```python
from build123d import *

# Parameters (mm, degrees)
BOSS_EXTRUDE2_DEPTH = 15
SKETCH5_R           = 1.5
CUT_EXTRUDE3_DEPTH  = 8
BOSS_EXTRUDE4_DEPTH = 5.5
CUT_EXTRUDE4_DEPTH  = 10
CUT_EXTRUDE5_DEPTH  = 7
SKETCH5_4_R         = 1.5
CUT_EXTRUDE6_DEPTH  = 10
SKETCH10_W          = 5.6
SKETCH10_H          = 2.4
SKETCH10_W_2        = 5.5
CUT_EXTRUDE7_DEPTH  = 24
SKETCH10_3_W        = 5.6
SKETCH10_3_H        = 2.4
SKETCH10_3_W_2      = 5.5
BOSS_EXTRUDE5_DEPTH = 4.2


with BuildPart() as part:
    # Sketch3 → Boss-Extrude2 (new body)
    with BuildSketch(Plane.XY):
        Polygon((380.706426849, -77.512840587), (380.706426849, -131.012840587), (354.706426849, -131.012840587), (337.706426849, -77.512840587), align=None)
    extrude(amount=BOSS_EXTRUDE2_DEPTH)

    # Sketch5 → Cut-Extrude3 (cut)
    with BuildSketch(Plane(origin=(0, -77.512840587, 0), x_dir=(1, 0, 0), z_dir=(0, 1, 0))):
        with Locations(Location((344.406426849, -7.5, 0), (0, 0, 270))):
            Circle(SKETCH5_R)
        with Locations(Location((359.406426849, -7.5, 0), (0, 0, 270))):
            Circle(SKETCH5_R)
        with Locations(Location((374.406426849, -7.5, 0), (0, 0, 270))):
            Circle(SKETCH5_R)
    extrude(amount=-CUT_EXTRUDE3_DEPTH, mode=Mode.SUBTRACT)

    # Sketch7 → Boss-Extrude4 (add)
    with BuildSketch(Plane(origin=(0, 0, 0), x_dir=(-1, 0, 0), z_dir=(0, 0, -1))):
        Polygon((-380.706426849, -77.512840587), (-337.706426849, -77.512840587), (-354.706426849, -131.012840587), (-380.706426849, -131.012840587), align=None)
    extrude(amount=BOSS_EXTRUDE4_DEPTH)

    # Sketch8 → Cut-Extrude4 (cut)
    with BuildSketch(Plane(origin=(380.706426849, 0, 0), x_dir=(0, 0, -1), z_dir=(1, 0, 0))):
        with BuildLine():
            ThreePointArc((-3.25, -98.312840587), (-3.689339828, -97.252180415), (-4.75, -96.812840587))
            Line((-4.75, -96.812840587), (-4.75, -99.812840587))
            ThreePointArc((-4.75, -99.812840587), (-3.689339828, -99.373500759), (-3.25, -98.312840587))
        make_face()
        with BuildLine():
            Line((-4.75, -99.812840587), (-4.75, -96.812840587))
            ThreePointArc((-4.75, -96.812840587), (-6.25, -98.312840587), (-4.75, -99.812840587))
        make_face()
        with BuildLine():
            ThreePointArc((-3.25, -122.312840587), (-3.689339828, -121.252180415), (-4.75, -120.812840587))
            Line((-4.75, -120.812840587), (-4.75, -123.812840587))
            ThreePointArc((-4.75, -123.812840587), (-3.689339828, -123.373500759), (-3.25, -122.312840587))
        make_face()
        with BuildLine():
            Line((-4.75, -123.812840587), (-4.75, -120.812840587))
            ThreePointArc((-4.75, -120.812840587), (-6.25, -122.312840587), (-4.75, -123.812840587))
        make_face()
    extrude(amount=-CUT_EXTRUDE4_DEPTH, mode=Mode.SUBTRACT)

    # Sketch9 → Cut-Extrude5 (cut)
    with BuildSketch(Plane(origin=(0, -131.012840587, 0), x_dir=(-1, 0, 0), z_dir=(0, -1, 0))):
        with BuildLine():
            ThreePointArc((-375.206426849, -4.75), (-373.706426849, -6.25), (-372.206426849, -4.75))
            Line((-372.206426849, -4.75), (-375.206426849, -4.75))
        make_face()
        with BuildLine():
            Line((-375.206426849, -4.75), (-372.206426849, -4.75))
            ThreePointArc((-372.206426849, -4.75), (-373.706426849, -3.25), (-375.206426849, -4.75))
        make_face()
        with BuildLine():
            ThreePointArc((-363.206426849, -4.75), (-361.706426849, -6.25), (-360.206426849, -4.75))
            Line((-360.206426849, -4.75), (-363.206426849, -4.75))
        make_face()
        with BuildLine():
            Line((-363.206426849, -4.75), (-360.206426849, -4.75))
            ThreePointArc((-360.206426849, -4.75), (-361.706426849, -3.25), (-363.206426849, -4.75))
        make_face()
    extrude(amount=-CUT_EXTRUDE5_DEPTH, mode=Mode.SUBTRACT)

    # Sketch5_4 → Cut-Extrude6 (cut)
    with BuildSketch(Plane(origin=(0, -77.512840587, 0), x_dir=(1, 0, 0), z_dir=(0, 1, 0))):
        with Locations(Location((359.406426849, -7.5, 0), (0, 0, 270))):
            Circle(SKETCH5_4_R)
        with Locations(Location((374.406426849, -7.5, 0), (0, 0, 270))):
            Circle(SKETCH5_4_R)
    extrude(amount=-CUT_EXTRUDE6_DEPTH, mode=Mode.SUBTRACT)

    # Sketch10 → Cut-Extrude7 (cut)
    with BuildSketch(Plane.XY.offset(15)):
        with Locations((359.312441298, -85.248108343)):
            Rectangle(SKETCH10_W, SKETCH10_H)
        with Locations((374.333669077, -85.248108343)):
            Rectangle(SKETCH10_W_2, SKETCH10_H)
    extrude(amount=-CUT_EXTRUDE7_DEPTH, mode=Mode.SUBTRACT)

    # Sketch10_3 → Boss-Extrude5 (add)
    with BuildSketch(Plane.XY.offset(15)):
        with Locations((359.312441298, -85.248108343)):
            Rectangle(SKETCH10_3_W, SKETCH10_3_H)
        with Locations((374.333669077, -85.248108343)):
            Rectangle(SKETCH10_3_W_2, SKETCH10_3_H)
    extrude(amount=-BOSS_EXTRUDE5_DEPTH)


solid = part.part
```
Geometry: final body of the model. Coordinates: model frame, mm. A direction names the side the tool comes from. Give positions to 0.01 mm unless a question says otherwise; leave off trailing zeros. Order: outer loops, then holes, each group sorted by start corner. A loop starts at its lowest first (then second) coordinate and runs counter-clockwise, first axis right, second up. Notation, with made-up numbers: M 35.5,40.25 L 46.5,40.25 A18 cw 46.5,49.25 Z; hole C 72.25,16.25 d9. An arc over 180 degrees is marked long. Answer as CSV lines item,"result". Start each with the question number.
1) Line query: line 1 (Y direction, x = 359, z = 10.5); line 2 (X direction, y = -126.25, z = 4.75); line 3 (X direction, y = -83, z = 7.5). Output: solid intervals per line, ascending. Write a range as from..to.
2) First-contact query: P1, Ø0.9, axis at x = 374, z = 5, coming from the -Y side. Flat tip, straight axial feed; report the tip coordinate or a pass-through.
3) Cut plane B-B (x = 376.5). Output: boundary loops of the cut face in (y, z).
4) Set-up query: faces 4 (the flat face through (344, -85.513, 7)), 5 (the cylindrical face through (375.205, -127.562, 4.684)), 6 (the flat face through (362.112, -85, 3)), 7 (the flat face through (370.706, -122, 5)). Return all of +Z, -Z, +X, -X, +Y, -Y with unobstructed straight access to the full face (end or side cutting, diameter ignored); none if empty.
5) Mould query, pull axis X, two halves, no side actions, for faces 1 (the flat face through (368, -131.013, 5)), 2 (the flat face through (370.706, -98, 5)), 3 (the cylindrical face through (372.942, -80.735, 7.175)). Classes: +X half, -X half, draft (parallel to the pull), parting line (faces both ways), or undercut.
6) Cut plane A-A (z = 0.5). Output: boundary loops of the cut face in (x, y), then the cut area to 3 significant figures.
7) Cut plane C-C (y = -81.5). Output: boundary loops of the cut face in (x, z), then the cut area to 3 significant figures.
Findings below:
1,line 1,"y = -131.01..-86.45, -84.05..-77.51"
1,line 2,"x = 353.19..360.21, 363.21..372.21, 375.21..380.71"
1,line 3,"x = 339.45..342.91, 345.91..357.91, 360.91..372.91, 375.91..380.71"
2,P1,"stops at y = -124.01"
3,outline,"M -131.01,-5.5 L -86.45,-5.5 L -86.45,10.8 L -84.05,10.8 L -84.05,-5.5 L -77.51,-5.5 L -77.51,15 L -131.01,15 Z; hole C -122.31,4.75 d3; hole C -98.31,4.75 d3"
4,face 4,"+Y"
4,face 5,"-Y"
4,face 6,"-Z"
4,face 7,"+X"
5,face 1,"draft"
5,face 2,"+X half"
5,face 3,"undercut"
6,outline,"M 337.71,-77.51 L 354.71,-131.01 L 380.71,-131.01 L 380.71,-77.51 Z; hole M 356.51,-86.45 L 362.11,-86.45 L 362.11,-84.05 L 356.51,-84.05 Z; hole M 371.58,-86.45 L 377.08,-86.45 L 377.08,-84.05 L 371.58,-84.05 Z"
6,area,"1,820 mm²"
7,outline,"M 338.97,-5.5 L 380.71,-5.5 L 380.71,15 L 338.97,15 Z; hole C 344.41,7.5 d3; hole C 359.41,7.5 d3; hole C 374.41,7.5 d3"
7,area,"834 mm²"
